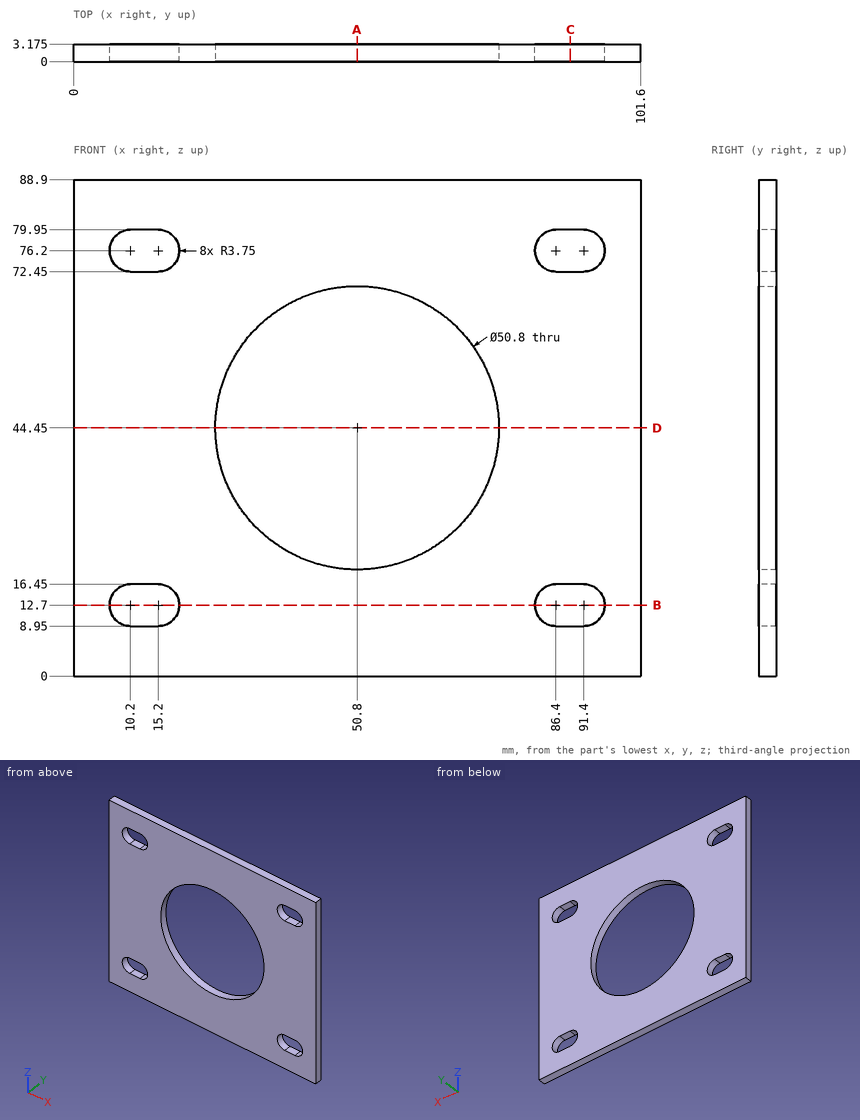
For this review, use the dimensioned drawing (mm, ordinates from the lowest corner) and the shaded views. Coordinates: 2 decimals unless noted, no trailing zeros. Order: outer loops, then holes, each group sorted by start corner. A loop starts at its lowest first (then second) coordinate and runs counter-clockwise, first axis right, second up. Notation, with made-up numbers: (37.5, 65) - (71.5, 65) arc R31 ccw to (71.5, 101) - close; hole circle Ø3 at (53, 66). An arc over 180 degrees is marked (long way). Answer as a JSON object with one key per item and string values. Group by question number.
1. We need section A-A on x = 50.8. State the section outline as (y, z) points (3 decimals).
2. We need section B-B on z = 12.7. State the section outline as (x, y) points (3 decimals).
3. We need section D-D on z = 44.45. State the section outline as (x, y) points (3 decimals).
4. We need section C-C on x = 89. State the section outline as (y, z) points (3 decimals).
5. For probe 1 along Z at (x, y) = (13.5, 0.7); probe 2 along X at (y, z) = (2.2, 44.45); probe 3 along X at (y, z) = (1.9, 15), list the stretches that pass through material, from the lowest coordinate up.
6. Clearance check with a flat-ended pin moving along its axis: P1, Ø1.6, axis at x = 89, y = 1.5, coming from the -Z side. State where the tip first meets the part, or that it passes through.
Final values:
{
 "1": {"outline": "(0, 0) - (3.175, 0) - (3.175, 19.05) - (0, 19.05) - close; (0, 69.85) - (3.175, 69.85) - (3.175, 88.9) - (0, 88.9) - close"},
 "2": {"outline": "(0, 0) - (6.45, 0) - (6.45, 3.175) - (0, 3.175) - close; (18.95, 0) - (82.65, 0) - (82.65, 3.175) - (18.95, 3.175) - close; (95.15, 0) - (101.6, 0) - (101.6, 3.175) - (95.15, 3.175) - close"},
 "3": {"outline": "(0, 0) - (25.4, 0) - (25.4, 3.175) - (0, 3.175) - close; (76.2, 0) - (101.6, 0) - (101.6, 3.175) - (76.2, 3.175) - close"},
 "4": {"outline": "(0, 0) - (3.175, 0) - (3.175, 8.95) - (0, 8.95) - close; (0, 16.45) - (3.175, 16.45) - (3.175, 72.45) - (0, 72.45) - close; (0, 79.95) - (3.175, 79.95) - (3.175, 88.9) - (0, 88.9) - close"},
 "5": {"probe 1": "0 to 8.95, 16.45 to 72.45, 79.95 to 88.9", "probe 2": "0 to 25.4, 76.2 to 101.6", "probe 3": "0 to 7.24, 18.16 to 83.44, 94.36 to 101.6"},
 "6": {"P1": "z = 0"}
}
